Autodesk Inventor part; units mm, degrees
ref_plane "YZ Plane" through (0, 0, 0) normal (1, 0, 0) x (0, 1, 0)
ref_plane "XZ Plane" through (0, 0, 0) normal (0, 1, 0) x (-1, 0, 0)
ref_plane "XY Plane" through (0, 0, 0) normal (0, 0, 1) x (1, 0, 0)
sketch "Sketch1" plane through (0, 0, 0) normal (0, 0, 1) x (1, 0, 0)
  circle A0 centre (0, 0) radius 3
  line L0 (-1.5, 2.5981) -> (-1.5, 3.4)
  line L1 (-1.5, 3.4) -> (1.5, 3.4)
  line L2 (1.5, 3.4) -> (1.5, 2.5981)
  line L3 (0, 4.68) -> (0, -4.28)
  line L4 (-4.2, 0) -> (4.2, 0)
  dimension "d0" = 6
  dimension "d1" = 3.4
  dimension "d2" = 3
extrude "Body" add sketch "Sketch1" against normal blind 5.35
sketch "Sketch2" plane through (0, 0, 0) normal (0, 0, 1) x (1, 0, 0)
  circle A0 centre (0, 0) radius 1.2
  dimension "d5" = 2.4
extrude "Face Boss" add sketch "Sketch2" along normal blind 0.3
sketch "Sketch3" plane through (0, 0, 0.3) normal (0, 0, 1) x (1, 0, 0)
  circle A0 centre (0, 0) radius 0.4
  dimension "d8" = 0.8
extrude "Extrusion3" add sketch "Sketch3" along normal blind 3
properties part number "Minebea_SMS6-20_StepperMotor_Mockup"
Model file for the job. Use its own axes, mm. A direction names the side the tool comes from. Coordinates: 2 decimals unless noted, no trailing zeros. Order: outer loops, then holes, each group sorted by start corner. A loop starts at its lowest first (then second) coordinate and runs counter-clockwise, first axis right, second up. Notation, with made-up numbers: (68.25, -32.75) - (86.25, -32.75) arc R27 ccw to (86.25, 4.25) - close; hole circle Ø1 at (-32.75, 51.5). An arc over 180 degrees is marked (long way). Return JSON: item names as keys, results as strings. Group by question number.
1) Flat gauge pins, fed straight in: P1, Ø2, axis at y = 2, z = -3, coming from the -X side; P2, Ø3, axis at y = -2, z = -1, coming from the -X side; P3, Ø2, axis at x = 1.5, y = 0.5, coming from the +Z side. Where does each tip first touch, or does it go through?
2) Saw through at C-C, the plane z = 0.5. Write the cut outline in (x, y), plus the area to 3 significant figures.
3) Tool access for faces 1 (the flat face through (-1.4, 0.2, 0)), 2 (the flat face through (0, 3.4, -3)), 3 (the flat face through (0, 0, -5.35)), 4 (the flat face through (-1.5, 3, -3)), 5 (the flat face through (1.5, 3, -3)): list every direction of +Z, -Z, +X, -X, +Y, -Y with a clear straight run to the whole face (end or side of a thin tool).
4) Saw through at B-B, the plane y = 0. Write the cut outline in (x, z), plus the area to 3 significant figures.
5) Probe line 1 (Z direction, x = 0.25, y = -1.25); line 2 (Y direction, x = 1.25, z = -1.75); line 3 (Y direction, x = 0.5, z = -1.25). List the from-to ranges inside material, lowest first. Write a range as from..to.
6) Saw through at D-D, the plane y = 1. Write the cut outline in (x, z), plus the area to 3 significant figures.
7) Saw through at A-A, the plane x = 0. Write the cut outline in (y, z), plus the area to 3 significant figures.
Values found:
{
 "1": {"P1": "stops at x = -2.83", "P2": "stops at x = -2.96", "P3": "stops at z = 0.3"},
 "2": {"outline": "circle Ø0.8 at (0, 0)", "area": "0.503 mm²"},
 "3": {"face 1": "+Z", "face 2": "+Z, -Z, +X, -X, +Y", "face 3": "-Z, +X, -X, +Y, -Y", "face 4": "+Z, -Z, -X, +Y", "face 5": "+Z, -Z, +X, +Y"},
 "4": {"outline": "(-3, -5.35) - (3, -5.35) - (3, 0) - (1.2, 0) - (1.2, 0.3) - (0.4, 0.3) - (0.4, 3.3) - (-0.4, 3.3) - (-0.4, 0.3) - (-1.2, 0.3) - (-1.2, 0) - (-3, 0) - close", "area": "35.2 mm²"},
 "5": {"line 1": "z = -5.35..0", "line 2": "y = -2.73..3.4", "line 3": "y = -2.96..3.4"},
 "6": {"outline": "(-2.83, -5.35) - (2.83, -5.35) - (2.83, 0) - (0.66, 0) - (0.66, 0.3) - (-0.66, 0.3) - (-0.66, 0) - (-2.83, 0) - close", "area": "30.7 mm²"},
 "7": {"outline": "(-3, -5.35) - (3.4, -5.35) - (3.4, 0) - (1.2, 0) - (1.2, 0.3) - (0.4, 0.3) - (0.4, 3.3) - (-0.4, 3.3) - (-0.4, 0.3) - (-1.2, 0.3) - (-1.2, 0) - (-3, 0) - close", "area": "37.4 mm²"}
}
